For this review, take the finished solid that the model builds, in its own axes (mm). Face numbers are marked on the shaded views. A direction names the side the tool comes from. Round coordinates to 2 decimals unless told otherwise and drop trailing zeros. Order: outer loops, then holes, each group sorted by start corner. A loop starts at its lowest first (then second) coordinate and runs counter-clockwise, first axis right, second up.
```python
from build123d import *

# Parameters (mm, degrees)
ESBO_O1_R                = 4
ESBO_O1_R_2              = 2.5
RESSALTO_EXTRUS_O1_DEPTH = 4
ESBO_O2_R                = 12.015701032
ESBO_O2_R_2              = 10.48384183
RESSALTO_EXTRUS_O2_DEPTH = 5
ESBO_O3_R                = 5.5
ESBO_O3_R_2              = 4
RESSALTO_EXTRUS_O3_DEPTH = 9
BOSS_EXTRUDE1_START      = -5
SKETCH1_R                = 13.5
BOSS_EXTRUDE1_DEPTH      = 5
SKETCH2_R                = 11
CUT_EXTRUDE1_DEPTH       = 7
CUT_EXTRUDE2_START       = -7
SKETCH3_R                = 5.5
CUT_EXTRUDE2_DEPTH       = 7


with BuildPart() as part:
    # Esboço1 → Ressalto-extrusão1 (new body)
    with BuildSketch(Plane.XY):
        with BuildLine():
            Line((-20.12399727, 5.170892982), (-8.093718556, 10.80470823))
            ThreePointArc((-8.093718556, 10.80470823), (0, 13.5), (8.093718556, 10.80470823))
            Line((8.093718556, 10.80470823), (20.12399727, 5.170892982))
            ThreePointArc((20.12399727, 5.170892982), (23.75, 0), (20.12399727, -5.170892982))
            Line((20.12399727, -5.170892982), (8.093718556, -10.80470823))
            ThreePointArc((8.093718556, -10.80470823), (0, -13.5), (-8.093718556, -10.80470823))
            Line((-8.093718556, -10.80470823), (-20.12399727, -5.170892982))
            ThreePointArc((-20.12399727, -5.170892982), (-23.75, 0), (-20.12399727, 5.170892982))
        make_face()
        Circle(ESBO_O1_R, mode=Mode.SUBTRACT)
        with Locations((-18.25, 0)):
            Circle(ESBO_O1_R_2, mode=Mode.SUBTRACT)
        with Locations((18.25, 0)):
            Circle(ESBO_O1_R_2, mode=Mode.SUBTRACT)
    extrude(amount=RESSALTO_EXTRUS_O1_DEPTH)

    # Esboço2 → Ressalto-extrusão2 (add)
    with BuildSketch(Plane.XY.offset(4)):
        Circle(ESBO_O2_R)
        Circle(ESBO_O2_R_2, mode=Mode.SUBTRACT)
    extrude(amount=RESSALTO_EXTRUS_O2_DEPTH)

    # Esboço3 → Ressalto-extrusão3 (add)
    with BuildSketch(Plane.XY.offset(4)):
        Circle(ESBO_O3_R)
        Circle(ESBO_O3_R_2, mode=Mode.SUBTRACT)
    extrude(amount=RESSALTO_EXTRUS_O3_DEPTH)

    # Sketch1 → Boss-Extrude1 (add)
    with BuildSketch(Plane.XY.offset(9).offset(BOSS_EXTRUDE1_START)):
        with Locations(Location((0, 0, 0), (0, 0, 126.836580816))):
            Circle(SKETCH1_R)
    extrude(amount=BOSS_EXTRUDE1_DEPTH)

    # Sketch2 → Cut-Extrude1 (cut)
    with BuildSketch(Plane(origin=(0, 0, 0), x_dir=(-1, 0, 0), z_dir=(0, 0, -1))):
        Circle(SKETCH2_R)
    extrude(amount=-CUT_EXTRUDE1_DEPTH, mode=Mode.SUBTRACT)

    # Sketch3 → Cut-Extrude2 (cut)
    with BuildSketch(Plane.XY.offset(13).offset(CUT_EXTRUDE2_START)):
        Circle(SKETCH3_R)
    extrude(amount=CUT_EXTRUDE2_DEPTH, mode=Mode.SUBTRACT)


solid = part.part
```
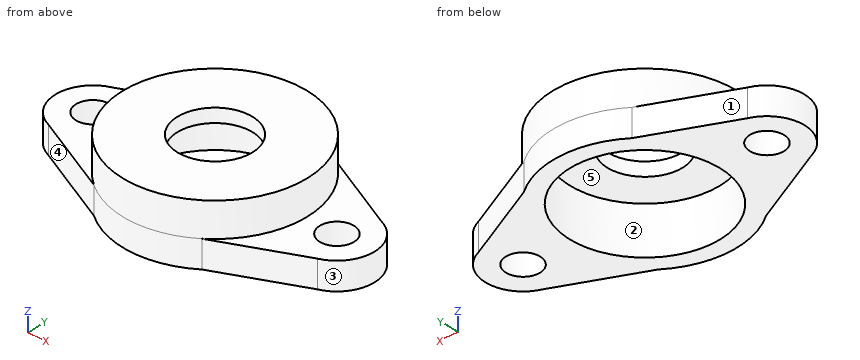
Q1. Tool access review of the marked faces 4 and 5: name each direction out of +Z, -Z, +X, -X, +Y, -Y from which nothing blocks a thin tool from reaching the whole face with its end or side.
Q2. Take a section at D-D, the plane y = -4. State the section outline as (x, z) points, plus the area to 3 significant figures.
Q3. Take a section at B-B, the plane x = 0. State the section outline as (y, z) points, plus the area to 3 significant figures.
Q4. Clearance check with flat-ended pins moving along their axes: pin 1 (4.5 mm diameter, centred on x = -18.25, y = 0, fed in from -Z); pin 2 (6 mm diameter, centred on x = 18.25, y = 0, fed in from +Z); pin 3 (1.5 mm diameter, centred on x = 9.5, z = 7.5, fed in from +Y); pin 4 (6.5 mm diameter, centred on x = -0.5, y = 3, fed in from -Z). State where each tip first meets the part, or that it passes through.
Q5. Take a section at A-A, the plane y = 0. State the section outline as (x, z) points, plus the area to 3 significant figures.
Q6. Mouldability with a two-part tool opening along X and no side actions: class the marked faces 1, 2 and 3 as +X half, -X half, draft (parallel to the pull), parting line (faces both ways), or undercut.
Q7. Wall thickness on line 1 (Y direction, x = 0, z = 3); line 2 (Y direction, x = 0, z = 8.35); line 3 (Z direction, x = 14.5, y = 1.25): over which ranges is each line inside the solid? List them lowest first.
Q8. Take a section at C-C, the plane z = 2. State the section outline as (x, y) points, plus the area to 3 significant figures.
Working result:
1. face 4: +Z, -Z, -X, -Y
1. face 5: -Z
2. outline: (-22.02, 0) - (-10.25, 0) - (-10.25, 7) - (-3.77, 7) - (-3.77, 9) - (-12.89, 9) - (-12.89, 4) - (-22.02, 4) - close; (3.77, 7) - (10.25, 7) - (10.25, 0) - (22.02, 0) - (22.02, 4) - (12.89, 4) - (12.89, 9) - (3.77, 9) - close
2. area: 147 mm2
3. outline: (-13.5, 0) - (-11, 0) - (-11, 7) - (-5.5, 7) - (-5.5, 9) - (-13.5, 9) - close; (5.5, 7) - (11, 7) - (11, 0) - (13.5, 0) - (13.5, 9) - (5.5, 9) - close
3. area: 67.0 mm2
4. pin 1: passes through
4. pin 2: stops at z = 4
4. pin 3: stops at y = 10.28
4. pin 4: stops at z = 7
5. outline: (-23.75, 0) - (-20.75, 0) - (-20.75, 4) - (-23.75, 4) - close; (-15.75, 0) - (-11, 0) - (-11, 7) - (-5.5, 7) - (-5.5, 9) - (-13.5, 9) - (-13.5, 4) - (-15.75, 4) - close; (5.5, 7) - (11, 7) - (11, 0) - (15.75, 0) - (15.75, 4) - (13.5, 4) - (13.5, 9) - (5.5, 9) - close; (20.75, 0) - (23.75, 0) - (23.75, 4) - (20.75, 4) - close
5. area: 109 mm2
6. face 1: -X half
6. face 2: undercut
6. face 3: +X half
7. line 1: y = -13.5 to -11, 11 to 13.5
7. line 2: y = -13.5 to -5.5, 5.5 to 13.5
7. line 3: z = 0 to 4
8. outline: (-20.12, -5.17) - (-8.09, -10.8) arc R13.5 ccw to (8.09, -10.8) - (20.12, -5.17) arc R5.5 ccw to (20.12, 5.17) - (8.09, 10.8) arc R13.5 ccw to (-8.09, 10.8) - (-20.12, 5.17) arc R5.5 ccw to start; hole circle Ø5 at (-18.25, 0); hole circle Ø22 at (0, 0); hole circle Ø5 at (18.25, 0)
8. area: 429 mm2
